Job drawing, mm, ordinate dimensions from the low corner. One solid piece. A direction names the side the tool comes from. Coordinates: 2 decimals unless noted, no trailing zeros. Order: outer loops, then holes, each group sorted by start corner. A loop starts at its lowest first (then second) coordinate and runs counter-clockwise, first axis right, second up. Notation, with made-up numbers: (3, 51) - (20, 51) arc R18 ccw to (20, 78) - close; hole circle Ø5 at (30, -24). An arc over 180 degrees is marked (long way). Use one line per item in the form item = value.
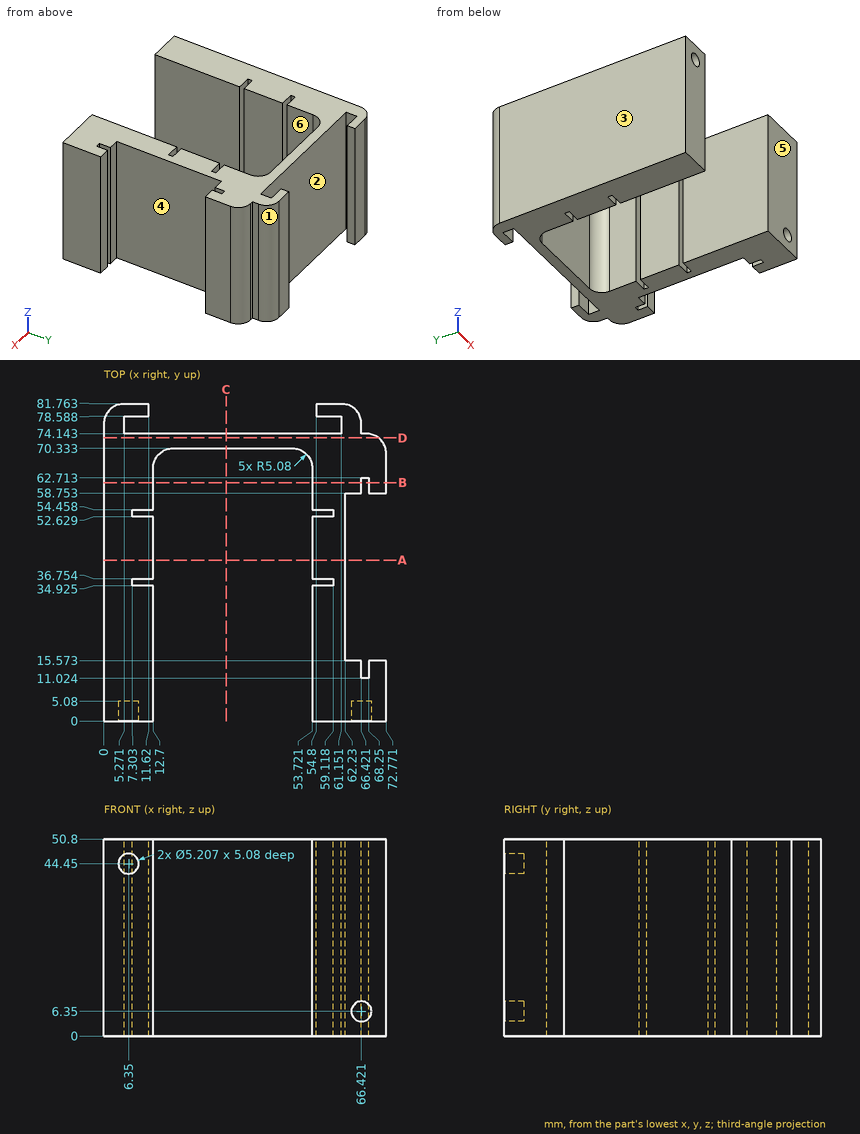
Item 1: Two-plate mould, pull along Y, no slides. Class the marked faces 1, 2 and 3: +Y half, -Y half, draft (parallel to the pull), parting line (faces both ways), or undercut.
Derived:
face_1 = +Y half
face_2 = undercut
face_3 = draft
Item 2: Cut at D-D, the plane y = 73. Write the cut outline in (x, z), plus the area to 3 significant figures.
Derived:
outline = (0, 0) - (70.9, 0) - (70.9, 50.8) - (0, 50.8) - close
area = 3,600 mm²
Item 3: Cut at B-B, the plane y = 61.5. Write the cut outline in (x, z), plus the area to 3 significant figures.
Derived:
outline = (0, 0) - (12.7, 0) - (12.7, 50.8) - (0, 50.8) - close; (53.72, 0) - (66.42, 0) - (66.42, 50.8) - (53.72, 50.8) - close; (68.25, 0) - (72.77, 0) - (72.77, 50.8) - (68.25, 50.8) - close
area = 1,520 mm²
Item 4: Cut at A-A, the plane y = 41.5. Write the cut outline in (x, z).
Derived:
outline = (0, 0) - (12.7, 0) - (12.7, 50.8) - (0, 50.8) - close; (53.72, 0) - (62.23, 0) - (62.23, 50.8) - (53.72, 50.8) - close
Item 5: Cut at C-C, the plane x = 31.5. Write the cut outline in (y, z).
Derived:
outline = (70.33, 0) - (74.14, 0) - (74.14, 50.8) - (70.33, 50.8) - close
Item 6: Drop flat-ended pins along their axis: pin 1 (4.5 mm diameter, centred on x = 64.5, z = 16, fed in from +Y); pin 2 (1.5 mm diameter, centred on x = 39, z = 16, fed in from -Y); pin 3 (3.5 mm diameter, centred on y = 77, z = 25, fed in from +X); pin 4 (5 mm diameter, centred on x = 25.5, y = 66, fed in from -Z). Give the stop position or say it passes through.
Derived:
pin_1 = 81.68
pin_2 = 70.33
pin_3 = 66.42
pin_4 = through
Item 7: Drill centre lines: line 1 (X direction, y = 59, z = 13); line 2 (Y direction, x = 10, z = 6) (1 decimal); line 3 (X direction, y = 75, z = 46). Where is each one in solid material? Low to high. Write a range as [from, to].
Derived:
line_1 = [0, 12.7], [53.72, 66.42], [68.25, 72.77]
line_2 = [0, 34.9], [36.8, 52.6], [54.5, 74.1], [78.6, 81.8]
line_3 = [0, 5.27], [61.15, 66.42]
Item 8: 3-axis set-ups, long thin cutter, end or side, ignore diameter. For the marked faces 4, 5 and 6: which of +Z, -Z, +X, -X, +Y, -Y reach the whole face in a straight line?
Derived:
face_4 = +Z, -Z, +X
face_5 = +Z, -Z, +X, -X, -Y
face_6 = +Z, -Z, -Y
